```python
from build123d import *

# Parameters (mm, degrees)
F1_DEPTH = 6.35
F2_R     = 7.9375
F2_R_2   = 3.175
F3_DEPTH = 6.35
F4_R     = 12.7
F5_DEPTH = 6.35
F6_DEPTH = 9.525


with BuildPart() as f1:
    # F0 (on Top) → F1 (new body)
    with BuildSketch(Plane.XY):
        with BuildLine():
            Line((-31.6207525557, -18.25625), (0, 0))
            Line((0, 0), (0, 36.5125))
            ThreePointArc((0, 36.5125), (-6.8740766425, 40.48125), (-6.8740766425, 48.41875))
            Line((-6.8740766425, 48.41875), (-21.9970452561, 57.15))
            Line((-21.9970452561, 57.15), (-60.4918744543, -9.525))
            Line((-60.4918744543, -9.525), (-45.3689058408, -18.25625))
            ThreePointArc((-45.3689058408, -18.25625), (-38.4948291982, -14.2875), (-31.6207525557, -18.25625))
        make_face()
        with BuildLine():
            ThreePointArc((-38.4948291982, -30.1625), (-45.3689058408, -26.19375), (-45.3689058408, -18.25625))
            Line((-45.3689058408, -18.25625), (-60.4918744543, -9.525))
            ThreePointArc((-60.4918744543, -9.525), (-60.4918744543, -34.925), (-38.4948291982, -47.625))
            Line((-38.4948291982, -47.625), (-38.4948291982, -30.1625))
        make_face()
        with BuildLine():
            Line((31.6207525557, -18.25625), (0, 0))
            Line((0, 0), (-31.6207525557, -18.25625))
            ThreePointArc((-31.6207525557, -18.25625), (-30.827792952, -20.1706238295), (-30.5573291982, -22.225))
            ThreePointArc((-30.5573291982, -22.225), (-32.8821691226, -27.8376600757), (-38.4948291982, -30.1625))
            Line((-38.4948291982, -30.1625), (-38.4948291982, -47.625))
            Line((-38.4948291982, -47.625), (38.4948291982, -47.625))
            Line((38.4948291982, -47.625), (38.4948291982, -30.1625))
            ThreePointArc((38.4948291982, -30.1625), (31.6207525557, -26.19375), (31.6207525557, -18.25625))
        make_face()
        with BuildLine():
            Line((60.4918744543, -9.525), (45.3689058408, -18.25625))
            ThreePointArc((45.3689058408, -18.25625), (46.1618654444, -20.1706238295), (46.4323291982, -22.225))
            ThreePointArc((46.4323291982, -22.225), (44.1074892739, -27.8376600757), (38.4948291982, -30.1625))
            Line((38.4948291982, -30.1625), (38.4948291982, -47.625))
            ThreePointArc((38.4948291982, -47.625), (60.4918744543, -34.925), (60.4918744543, -9.525))
        make_face()
        with BuildLine():
            Line((0, 36.5125), (0, 0))
            Line((0, 0), (31.6207525557, -18.25625))
            ThreePointArc((31.6207525557, -18.25625), (38.4948291982, -14.2875), (45.3689058408, -18.25625))
            Line((45.3689058408, -18.25625), (60.4918744543, -9.525))
            Line((60.4918744543, -9.525), (21.9970452561, 57.15))
            Line((21.9970452561, 57.15), (6.8740766425, 48.41875))
            ThreePointArc((6.8740766425, 48.41875), (7.6670362462, 46.5043761705), (7.9375, 44.45))
            ThreePointArc((7.9375, 44.45), (5.6126600757, 38.8373399243), (0, 36.5125))
        make_face()
        with BuildLine():
            Line((-21.9970452561, 57.15), (-6.8740766425, 48.41875))
            ThreePointArc((-6.8740766425, 48.41875), (0, 52.3875), (6.8740766425, 48.41875))
            Line((6.8740766425, 48.41875), (21.9970452561, 57.15))
            ThreePointArc((21.9970452561, 57.15), (0, 69.85), (-21.9970452561, 57.15))
        make_face()
    extrude(amount=F1_DEPTH)

    # F2 (on face) → F3 (join)
    with BuildSketch(Plane(origin=(0, 0, 0), x_dir=(1, 0, 0), z_dir=(0, 0, -1))):
        with BuildLine():
            ThreePointArc((-38.4948291982, 47.625), (-60.4918744543, 34.925), (-60.4918744543, 9.525))
            Line((-60.4918744543, 9.525), (-21.9970452561, -57.15))
            ThreePointArc((-21.9970452561, -57.15), (0, -69.85), (21.9970452561, -57.15))
            Line((21.9970452561, -57.15), (60.4918744543, 9.525))
            ThreePointArc((60.4918744543, 9.525), (60.4918744543, 34.925), (38.4948291982, 47.625))
            Line((38.4948291982, 47.625), (-38.4948291982, 47.625))
        make_face()
        with Locations((0, -44.45)):
            Circle(F2_R, mode=Mode.SUBTRACT)
        with Locations((-38.4948291982, 22.225)):
            Circle(F2_R, mode=Mode.SUBTRACT)
        with Locations((38.4948291982, 22.225)):
            Circle(F2_R, mode=Mode.SUBTRACT)
        with Locations((0, -44.45)):
            Circle(F2_R)
        with Locations((0, -44.45)):
            Circle(F2_R_2, mode=Mode.SUBTRACT)
        with Locations((38.4948291982, 22.225)):
            Circle(F2_R)
        with Locations((38.4948291982, 22.225)):
            Circle(F2_R_2, mode=Mode.SUBTRACT)
        with Locations((-38.4948291982, 22.225)):
            Circle(F2_R)
        with Locations((-38.4948291982, 22.225)):
            Circle(F2_R_2, mode=Mode.SUBTRACT)
    extrude(amount=F3_DEPTH)

    # F4 (on face) → F5 (cut)
    with BuildSketch(Plane.XY.offset(6.35)):
        with BuildLine():
            ThreePointArc((21.9970452561, 57.15), (0, 69.85), (-21.9970452561, 57.15))
            Line((-21.9970452561, 57.15), (-60.4918744543, -9.525))
            ThreePointArc((-60.4918744543, -9.525), (-60.4918744543, -34.925), (-38.4948291982, -47.625))
            Line((-38.4948291982, -47.625), (38.4948291982, -47.625))
            ThreePointArc((38.4948291982, -47.625), (60.4918744543, -34.925), (60.4918744543, -9.525))
            Line((60.4918744543, -9.525), (21.9970452561, 57.15))
        make_face()
        with Locations((-38.4948291982, -22.225)):
            Circle(F4_R, mode=Mode.SUBTRACT)
        with Locations((38.4948291982, -22.225)):
            Circle(F4_R, mode=Mode.SUBTRACT)
        with Locations((0, 44.45)):
            Circle(F4_R, mode=Mode.SUBTRACT)
    extrude(amount=-F5_DEPTH, mode=Mode.SUBTRACT)

    # F6 (add): faces of the model
    f6_faces = [f1.faces().sort_by_distance(p)[0] for p in [
        (-50.8356189534, -22.225, 6.35),
        (-12.3407897552, 44.45, 6.35),
        (26.1540394431, -22.225, 6.35),
    ]]
    extrude(f6_faces, amount=F6_DEPTH)


solid = f1.part
```
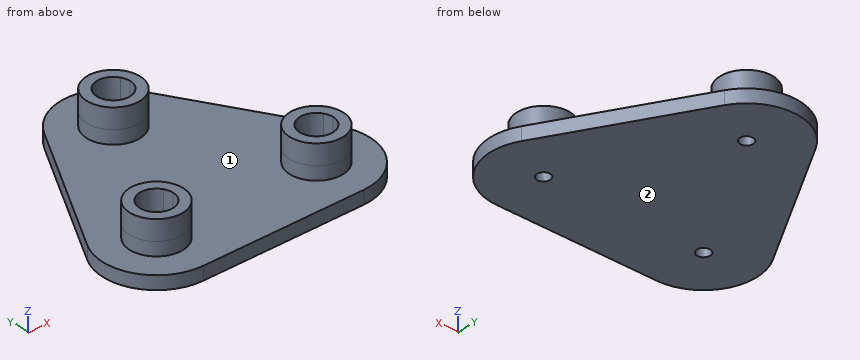
Source: CAD feature listing. Evaluate the final solid. Frame: model axes, mm. Face numbers are marked on the shaded views. Round coordinates to 2 decimals unless told otherwise and drop trailing zeros. Loops run counter-clockwise (first coordinate to the right, second up) from the corner with the lowest first, then second, coordinate; pieces in that order, holes last.
1. Section query D-D on z = -4.25. Output: boundary loops of the cut face in (x, y) (3 decimals).
2. Section query B-B on y = -24. Output: boundary loops of the cut face in (x, z) (3 decimals), and give its area (3 significant figures).
3. Ray query, L1, parallel to Y at x = 0, z = -1.75 (3 decimals); L2, parallel to X at y = -17.5, z = 4.75; L3, parallel to Z at x = 25.5, y = -6. Return the intervals inside material, ascending.
4. Mould query, pull axis X, two halves, no side actions, for the marked faces 1 and 2. Classes: released by +X, released by -X, zero draft, split by the parting line, or undercut.
5. Section query C-C on x = -37. Output: boundary loops of the cut face in (y, z) (3 decimals), and give its area (3 significant figures).
6. Section query A-A on z = 9.25. Give the number of separate pieces and of enclosed holes in the cut face, and give its area (3 significant figures).
7. Contact query for flat-ended pins moving along their axis: pin 1 (5 mm diameter, centred on y = -17.5, z = 10, fed in from +X); pin 2 (1.5 mm diameter, centred on y = 46, z = -4, fed in from +X); pin 3 (5 mm diameter, centred on x = 6.5, z = 13, fed in from +Y). Output: stop coordinate, or through.
Answers below:
1. outline: (-60.492, -9.525) arc R25.4 ccw to (-38.495, -47.625) - (38.495, -47.625) arc R25.4 ccw to (60.492, -9.525) - (21.997, 57.15) arc R25.4 ccw to (-21.997, 57.15) - close; hole circle Ø6.35 at (-38.495, -22.225); hole circle Ø6.35 at (0, 44.45); hole circle Ø6.35 at (38.495, -22.225)
2. outline: (-63.833, -6.35) - (-41.127, -6.35) - (-41.127, 0) - (-46.231, 0) - (-46.231, 15.875) - (-51.07, 15.875) - (-51.07, 0) - (-63.833, 0) - close; (-35.862, -6.35) - (35.862, -6.35) - (35.862, 0) - (30.758, 0) - (30.758, 15.875) - (25.919, 15.875) - (25.919, 0) - (-25.919, 0) - (-25.919, 15.875) - (-30.758, 15.875) - (-30.758, 0) - (-35.862, 0) - close; (41.127, -6.35) - (63.833, -6.35) - (63.833, 0) - (51.07, 0) - (51.07, 15.875) - (46.231, 15.875) - (46.231, 0) - (41.127, 0) - close
2. area: 1,050 mm2
3. L1: y = -47.625 to 41.275, 47.625 to 69.85
3. L2: x = -50.28 to -44.87, -32.12 to -26.71, 26.71 to 32.12, 44.87 to 50.28
3. L3: z = -6.35 to 0
4. face 1: undercut
4. face 2: zero draft
5. outline: (-47.625, -6.35) - (-25.026, -6.35) - (-25.026, 0) - (-30.02, 0) - (-30.02, 15.875) - (-34.837, 15.875) - (-34.837, 0) - (-47.625, 0) - close; (-19.424, -6.35) - (31.164, -6.35) - (31.164, 0) - (-9.613, 0) - (-9.613, 15.875) - (-14.43, 15.875) - (-14.43, 0) - (-19.424, 0) - close
5. area: 618 mm2
6. separate pieces: 3
6. enclosed holes: 3
6. area: 926 mm2
7. pin 1: stops at x = 51
7. pin 2: stops at x = 28.87
7. pin 3: stops at y = 56.5
